Verification items for the finished model (mm, model axes). A direction names the side the tool comes from. Give positions to 0.01 mm unless a question says otherwise; leave off trailing zeros. Loops run counter-clockwise (first coordinate to the right, second up) from the corner with the lowest first, then second, coordinate; pieces in that order, holes last. Notation, with made-up numbers: (35.25, 79.25) - (69.25, 79.25) arc R25 ccw to (69.25, 112.25) - close; hole circle Ø7 at (87, 5). An arc over 180 degrees is marked (long way). One line per item, written item: value. Start each with the question number.
1. Scan lines: L1, parallel to X at y = 0.25, z = -6.75; L2, parallel to X at y = 3.5, z = -4.25; L3, parallel to X at y = -1.5, z = -1. Record each from-to range of solid material in increasing order. Write a range as [from, to].
2. Sectioned sample at A-A (y = -9). Record the cut outline in (x, z).
3. Sectioned sample at C-C (z = -6.5). Record the cut outline in (x, y).
4. Mould release check, pull along X, two halves, no side actions. Record for faces 1 (the cylindrical face through (10, 3.2, -3.7)), 2 (the flat face through (9, -0.5, -4)), 3 (the flat face through (-9, 0, -2.5)), 4 (the flat face through (-5, -9, 0)): pulls with the +X half, pulls with the -X half, needs draft (parallel to the pull), parting line crosses it, or undercut.
5. Access from +Z, -Z, +X, -X, +Y, -Y to the whole of each face (thin tool, end or side, straight path). Record for faces 5 (the flat face through (-9, 0, -5.5)), 6 (the flat face through (9, 0, -2.5)), 7 (the flat face through (-0.5, -9, -4)).
6. Gauge pin test, flat ends, axial feed: pin 1 (6.5 mm diameter, centred on x = 0, y = 0, fed in from -Z); pin 2 (1 mm diameter, centred on y = -2, z = -5.5, fed in from -X); pin 3 (1.1 mm diameter, centred on y = 9, z = -4, fed in from +X). Record the tip position at first contact, or that the pin passes through.
7. Sectioned sample at D-D (z = -2). Count the separate pieces of the cut face and the enclosed holes in it, plus the area to 3 significant figures.
from build123d import *

# Parameters (mm, degrees)
F0_R      = 10.5
F0_R_2    = 9.5
F1_DEPTH  = 7.5
F0_R_3    = 8.5
F0_R_4    = 3.5
F2_DEPTH  = 6
F5_W      = 9
F5_H      = 1
F5_W_2    = 1
F5_H_2    = 9
F6_DEPTH  = 3
F8_R      = 3.5
F8_R_2    = 1.5
F9_DEPTH  = 3.5
F0_R_5    = 1.5
F10_DEPTH = 6


with BuildPart() as f1:
    # F0 (on Top) → F1 (new body)
    with BuildSketch(Plane.XY):
        Circle(F0_R)
        Circle(F0_R_2, mode=Mode.SUBTRACT)
    extrude(amount=-F1_DEPTH)



with BuildPart() as f2:
    # F0 (on Top) → F2 (new body)
    with BuildSketch(Plane.XY):
        Circle(F0_R_3)
        Circle(F0_R_4, mode=Mode.SUBTRACT)
    extrude(amount=-F2_DEPTH)


with BuildPart() as f1_1:
    add(f1.part)

    add(f2.part)  # F6 merges F2
    # F5 (on offset) → F6 (join)
    with BuildSketch(Plane.XY.offset(-2.5)):
        with Locations((-5, 0)):
            Rectangle(F5_W, F5_H)
        with Locations((0, 5)):
            Rectangle(F5_W_2, F5_H_2)
        Rectangle(F5_W_2, F5_H)
        with Locations((5, 0)):
            Rectangle(F5_W, F5_H)
        with Locations((0, -5)):
            Rectangle(F5_W_2, F5_H_2)
    extrude(amount=-F6_DEPTH)

    # F3 (on Front) → F7 (revolve, cut)
    with BuildSketch(Plane.XZ):
        with BuildLine():
            Line((0, 0.069658272), (-8.4977783263, 0.0271935514))
            add(Edge.make_bspline(
                [(-8.4977783263, 0.0271935514), (-8.4390711904, -0.1936509699), (-8.5319644113, -0.9331612071), (-7.3101581266, -2.5228604066), (-4.8192842499, -3.2569469358), (-3.4470196357, -1.6163358317), (-2.5980696171, -0.2120298583), (-0.5223557571, -0.492685907), (0, -0.1791804971)],
                knots=[0, 0, 0, 0, 0.1159478411, 0.2887836686, 0.4788440423, 0.6507860288, 0.8064986974, 1, 1, 1, 1], degree=3))
            Line((0, -0.1791804971), (0, 0.069658272))
        make_face()
    revolve(axis=Axis((0, 0, 0.069658272), (0, 0, -1)), mode=Mode.SUBTRACT)

    # F8 (on offset) → F9 (join, through all)
    with BuildSketch(Plane.XY.offset(-2.5)):
        Circle(F8_R)
        Circle(F8_R_2, mode=Mode.SUBTRACT)
    extrude(amount=-F9_DEPTH)

    # F0 (on Top) → F10 (cut, through all)
    with BuildSketch(Plane.XY):
        Circle(F0_R_5)
    extrude(amount=-F10_DEPTH, mode=Mode.SUBTRACT)


solid = f1_1.part
Results are:
1. L1: x = [-10.5, -9.5], [9.5, 10.5]
1. L2: x = [-9.9, -8.83], [-7.75, 7.75], [8.83, 9.9]
1. L3: x = [-10.39, -9.38], [-8.37, -8.18], [8.18, 8.37], [9.38, 10.39]
2. outline: (-5.41, -7.5) - (-3.04, -7.5) - (-3.04, 0) - (-5.41, 0) - close; (-0.5, -5.5) - (0.5, -5.5) - (0.5, -2.5) - (-0.5, -2.5) - close; (3.04, -7.5) - (5.41, -7.5) - (5.41, 0) - (3.04, 0) - close
3. outline: circle Ø21 at (0, 0); hole circle Ø19 at (0, 0)
4. face 1: parting line crosses it
4. face 2: undercut
4. face 3: undercut
4. face 4: needs draft
5. face 5: -Z
5. face 6: +Z
5. face 7: +Z, -Z
6. pin 1: stops at z = -6
6. pin 2: stops at x = -10.39
6. pin 3: stops at x = 6.23
7. separate pieces: 3
7. enclosed holes: 3
7. area: 117 mm^2
